```python
from build123d import *

# Parameters (mm, degrees)
SKETCH1_W           = 140
SKETCH1_H           = 100
BOSS_EXTRUDE2_DEPTH = 40
BOSS_EXTRUDE2_TAPER = 20
SHELL1_T            = -5
SKETCH3_R           = 3.25
SKETCH3_W           = 80
SKETCH3_H           = 30
CUT_EXTRUDE1_DEPTH  = 95.868329974


with BuildPart() as part:
    # Sketch1 → Boss-Extrude2 (new body)
    with BuildSketch(Plane(origin=(0, 0, 0), x_dir=(1, 0, 0), z_dir=(0, 1, 0))):
        Rectangle(SKETCH1_W, SKETCH1_H)
    extrude(amount=BOSS_EXTRUDE2_DEPTH, taper=BOSS_EXTRUDE2_TAPER)

    # Shell1
    shell1_openings = [part.faces().sort_by_distance(p)[0] for p in [
        (0, 0, 0),
    ]]
    offset(amount=SHELL1_T, openings=shell1_openings, kind=Kind.INTERSECTION)

    # Sketch3 → Cut-Extrude1 (cut, through all)
    with BuildSketch(Plane(origin=(0, 40, 0), x_dir=(1, 0, 0), z_dir=(0, 1, 0))):
        with Locations(Location((0, -23.631190629, 0), (0, 0, 270))):
            Circle(SKETCH3_R)
        with Locations(Location((-27.720595315, 23.631190629, 0), (0, 0, 270))):
            Circle(SKETCH3_R)
        with Locations(Location((27.720595315, 23.631190629, 0), (0, 0, 270))):
            Circle(SKETCH3_R)
        Rectangle(SKETCH3_W, SKETCH3_H)
    extrude(amount=-CUT_EXTRUDE1_DEPTH, mode=Mode.SUBTRACT)


solid = part.part
```
Design review of the part built by this model. Coordinates are the model's own, in mm. A direction names the side the tool comes from. Coordinates: 2 decimals unless noted, no trailing zeros.
1) To check wall thickness, follow L1, parallel to X at y = 3, z = -18; L2, parallel to X at y = 34.5, z = -17.5; L3, parallel to Z at x = -52.5, y = 9.5. State the ranges of each line that lie inside material, in increasing order.
2) Machinability: for faces 3 (the flat face through (-10, 0, -46)), 4 (the flat face through (-40, 38, 0)), which of the approach directions +Z, -Z, +X, -X, +Y, -Y give a long, thin tool a straight path to every point of the face, cutting with its end or side? Answer none if there is none.
3) Insertion check: pin 1 (10 mm diameter, centred on y = 22.5, z = -30.5, fed in from +X); pin 2 (4 mm diameter, centred on x = -23, z = -16, fed in from -Y); pin 3 (1.5 mm diameter, centred on x = 7, y = 36.5, fed in from -Z). Each pin has a flat end and moves straight along its axis. Give the tip position at first contact, or say it passes through.
4) Add section A-A (x = 0). State how many separate pieces and enclosed holes the cut face has, plus the area to 3 significant figures.
5) Mouldability with a two-part tool opening along X and no side actions: class faces 1 (the flat face through (-1, 35, 16)), 2 (the flat face through (9.4, 40, 15.3)) as +X half, -X half, draft (parallel to the pull), parting line (faces both ways), or undercut.
Check result:
1. L1: x = -68.91 to -63.59, 63.59 to 68.91
1. L2: x = -57.44 to -52.12, 52.12 to 57.44
1. L3: z = -46.54 to -41.22, 41.22 to 46.54
2. face 3: +Z, -Z, +X, -X, -Y
2. face 4: +Y, -Y
3. pin 1: stops at x = 63.63
3. pin 2: stops at y = 35
3. pin 3: stops at z = -36.99
4. separate pieces: 3
4. enclosed holes: 0
4. area: 553 mm2
5. face 1: undercut
5. face 2: draft
